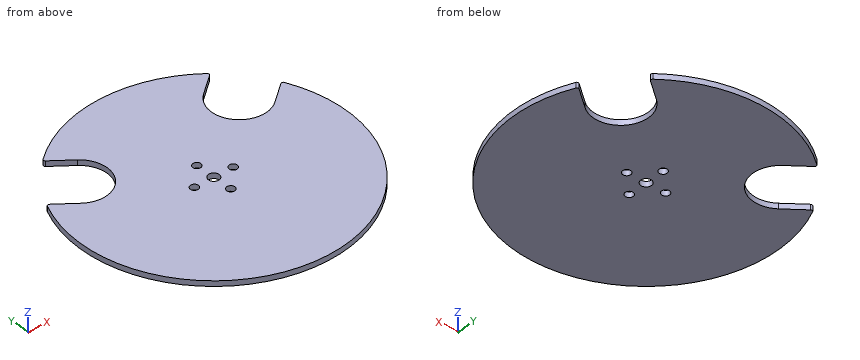
```python
from build123d import *

# Parameters (mm, degrees)
ESQUISSE1_R        = 2.25
ESQUISSE1_R_2      = 3
BOSS_EXTRU_1_DEPTH = 3
CONG_3_R           = 1


with BuildPart() as part:
    # Esquisse1 → Boss.-Extru.1 (new body)
    with BuildSketch(Plane.XY):
        with BuildLine():
            Line((66.562015248, 32.334163451), (54.8533712, 23.18636815))
            ThreePointArc((54.8533712, 23.18636815), (33.096451651, 25.857781964), (35.767865465, 47.614701512))
            Line((35.767865465, 47.614701512), (47.476509513, 56.762496813))
            ThreePointArc((47.476509513, 56.762496813), (0, 74), (-47.476509513, 56.762496813))
            Line((-47.476509513, 56.762496813), (-35.767865465, 47.614701512))
            ThreePointArc((-35.767865465, 47.614701512), (-33.096451651, 25.857781964), (-54.8533712, 23.18636815))
            Line((-54.8533712, 23.18636815), (-66.562015248, 32.334163451))
            ThreePointArc((-66.562015248, 32.334163451), (0, -74), (66.562015248, 32.334163451))
        make_face()
        with Locations((0, 11)):
            Circle(ESQUISSE1_R, mode=Mode.SUBTRACT)
        with Locations((11, 0)):
            Circle(ESQUISSE1_R, mode=Mode.SUBTRACT)
        with Locations((0, -11)):
            Circle(ESQUISSE1_R, mode=Mode.SUBTRACT)
        with Locations((-11, 0)):
            Circle(ESQUISSE1_R, mode=Mode.SUBTRACT)
        Circle(ESQUISSE1_R_2, mode=Mode.SUBTRACT)
    extrude(amount=BOSS_EXTRU_1_DEPTH)

    # Congé3
    cong_3_edges = [part.edges().sort_by_distance(p)[0] for p in [
        (-66.562015248, 32.334163451, 1.5),
        (-47.476509513, 56.762496813, 1.5),
        (47.476509513, 56.762496813, 1.5),
        (66.562015248, 32.334163451, 1.5),
    ]]
    fillet(cong_3_edges, radius=CONG_3_R)


solid = part.part
```
Check sheet for the modelled part. Datum: model origin and axes. Units: mm. Coordinates: 2 decimals unless noted, no trailing zeros. Loops run counter-clockwise (first coordinate to the right, second up) from the corner with the lowest first, then second, coordinate; pieces in that order, holes last.
1) Gauge pin test, flat ends, axial feed: pin 1 (1 mm diameter, centred on y = 42, z = 2, fed in from +X); pin 2 (1.5 mm diameter, centred on x = 8, z = 1, fed in from +Y). Record the tip position at first contact, or that the pin passes through.
2) Sectioned sample at D-D (x = -40). Record the boundary of the cut face in (y, z), and give its area (3 significant figures).
3) Sectioned sample at A-A (x = 0). Record the boundary of the cut face in (y, z), and give its area (3 significant figures).
4) Material ranges on probe 1 along Y at (x, z) = (0, 1.5); probe 2 along X at (y, z) = (-1.5, 1.4); probe 3 along X at (y, z) = (22, 1.4), recorded low to high.
5) Sectioned sample at C-C (z = 1.4). Record the boundary of the cut face in (x, y).
6) Sectioned sample at B-B (y = 27). Record the boundary of the cut face in (x, z), and give its area (3 significant figures).
Check sheet entries:
1. pin 1: stops at x = 31.53
1. pin 2: stops at y = 73.64
2. outline: (-62.26, 0) - (20.84, 0) - (20.84, 3) - (-62.26, 3) - close; (50.92, 0) - (62.26, 0) - (62.26, 3) - (50.92, 3) - close
2. area: 283 mm2
3. outline: (-74, 0) - (-13.25, 0) - (-13.25, 3) - (-74, 3) - close; (-8.75, 0) - (-3, 0) - (-3, 3) - (-8.75, 3) - close; (3, 0) - (8.75, 0) - (8.75, 3) - (3, 3) - close; (13.25, 0) - (74, 0) - (74, 3) - (13.25, 3) - close
3. area: 399 mm2
4. probe 1: y = -74 to -13.25, -8.75 to -3, 3 to 8.75, 13.25 to 74
4. probe 2: x = -73.98 to -12.68, -9.32 to -2.6, 2.6 to 9.32, 12.68 to 73.98
4. probe 3: x = -70.65 to -53.1, -37.52 to 37.52, 53.1 to 70.65
5. outline: (-67.1, 31.2) arc R74 ccw (long way) to (67.1, 31.2) arc R1 ccw to (65.58, 31.57) - (54.85, 23.19) arc R15.5 cw to (35.77, 47.61) - (46.49, 55.99) arc R1 ccw to (46.51, 57.56) arc R74 ccw to (-46.51, 57.56) arc R1 ccw to (-46.49, 55.99) - (-35.77, 47.61) arc R15.5 cw to (-54.85, 23.19) - (-65.58, 31.57) arc R1 ccw to start; hole circle Ø4.5 at (-11, 0); hole circle Ø6 at (0, 0); hole circle Ø4.5 at (0, -11); hole circle Ø4.5 at (0, 11); hole circle Ø4.5 at (11, 0)
6. outline: (-68.9, 0) - (-59.73, 0) - (-59.73, 3) - (-68.9, 3) - close; (-32.28, 0) - (32.28, 0) - (32.28, 3) - (-32.28, 3) - close; (59.73, 0) - (68.9, 0) - (68.9, 3) - (59.73, 3) - close
6. area: 249 mm2
